Can you work these out from the model? Positions are in its coordinate system, mm. A direction names the side the tool comes from. Give positions to 0.01 mm unless a question says otherwise; leave off trailing zeros. Loops run counter-clockwise (first coordinate to the right, second up) from the corner with the lowest first, then second, coordinate; pieces in that order, holes last. Notation, with made-up numbers: M 74,74.25 L 126,74.25 A29 ccw 126,107.25 Z; hole C 51,84 d9. An arc over 180 degrees is marked long. Answer as a JSON object with one key per item and string values.
```python
from build123d import *

# Parameters (mm, degrees)
SKETCH1_R          = 3.175
EXTRUDE1_DEPTH     = 76.2
CHAMFER3_SIZE      = 0.9525
SKETCH6_R          = 4.7625
EXTRUDE2_DEPTH     = 6.35
CUT_EXTRUDE1_DEPTH = 3.571875
CHAMFER1_SIZE      = 0.47625
CHAMFER2_SIZE      = 0.238125


with BuildPart() as part:
    # Sketch1 → Extrude1 (new body)
    with BuildSketch(Plane.XY):
        Circle(SKETCH1_R)
    extrude(amount=-EXTRUDE1_DEPTH)

    # Chamfer3
    chamfer3_edges = [part.edges().sort_by_distance(p)[0] for p in [
        (-3.175, 0, 0),
    ]]
    chamfer(chamfer3_edges, length=CHAMFER3_SIZE)

    # Sketch6 → Extrude2 (add)
    with BuildSketch(Plane(origin=(0, 0, -76.2), x_dir=(-1, 0, 0), z_dir=(0, 0, -1))):
        Circle(SKETCH6_R)
    extrude(amount=EXTRUDE2_DEPTH)

    # Sketch7 → Cut-Extrude1 (cut)
    with BuildSketch(Plane(origin=(0, 0, -82.55), x_dir=(-1, 0, 0), z_dir=(0, 0, -1))):
        Polygon((0, 2.749630657), (-2.38125, 1.374815329), (-2.38125, -1.374815329), (0, -2.749630657), (2.38125, -1.374815329), (2.38125, 1.374815329), align=None)
    extrude(amount=-CUT_EXTRUDE1_DEPTH, mode=Mode.SUBTRACT)

    # Cut-Extrude2 cone 1 section (through the dimple's axis) → Cut-Extrude2 (revolve, cut)
    with BuildSketch(Plane(origin=(0, 0, -82.55), x_dir=(0, 1, 0), z_dir=(1, 0, 0))):
        Polygon((0, 0), (2.749630657, 0), (0, 2.749630657), align=None)
    revolve(axis=Axis((0, 0, -82.55), (0, 0, 1)), mode=Mode.SUBTRACT)

    # Chamfer1
    chamfer1_edges = [part.edges().sort_by_distance(p)[0] for p in [
        (4.7625, 0, -82.55),
    ]]
    chamfer(chamfer1_edges, length=CHAMFER1_SIZE)

    # Chamfer2
    chamfer2_edges = [part.edges().sort_by_distance(p)[0] for p in [
        (4.7625, 0, -76.2),
    ]]
    chamfer(chamfer2_edges, length=CHAMFER2_SIZE)


solid = part.part
```
1) If we mould it in two halves opening along X, with no side actions, what happens to faces 1 (the flat face through (0, 0, 0)), 2 (the flat face through (-1.174, -2.072, -80.789)), 3 (the cylindrical face through (-0.69, -3.1, -38.05))? For each: +X half, -X half, draft (parallel to the pull), parting line (faces both ways), or undercut.
Answer list:
{"face 1": "draft", "face 2": "undercut", "face 3": "parting line"}
2) Suppose I cut it at B-B, the plane z = -16. Write out the boundary of the cut face in (x, y) (3 decimals), and give its area (3 significant figures).
Answer list:
{"outline": "C 0,0 d6.35", "area": "31.7 mm^2"}
3) Please list where these lines run through material, in increasing order: line 1 along Z through (x, y) = (-4, -1.5); line 2 along Z through (x, y) = (0.5, -1); line 3 along X through (y, z) = (2.25, -71). Write a range as from..to.
Answer list:
{"line 1": "-82.55..-76.2", "line 2": "-78.98..0", "line 3": "-2.24..2.24"}
4) For faces 4 (the flat face through (1.174, 2.072, -80.789)), 5 (the flat face through (-2, -3, -76.2)), 6 (the flat face through (0, -3, -82.55)), which set-ups out of +Z, -Z, +X, -X, +Y, -Y let a thin tool reach every point of the face, with its end or its side?
Answer list:
{"face 4": "-Z", "face 5": "+Z", "face 6": "-Z, +X, -X, +Y, -Y"}
5) Will these pins go through, and if not, where does the flat tip stop? pin 1 Ø1.5 at (x, z) = (1.5, -41.5) entering from +Y; pin 2 Ø2 at (y, z) = (3, -9.5) entering from -X; pin 3 Ø4 at (x, z) = (3.5, -54.5) entering from +Y.
Answer list:
{"pin 1": "y = 3.09", "pin 2": "x = -2.47", "pin 3": "y = 2.8"}
